The model under review builds one solid part; all positions refer to its coordinate system, in mm. A direction names the side the tool comes from. Round coordinates to 2 decimals unless told otherwise and drop trailing zeros. Loops run counter-clockwise (first coordinate to the right, second up) from the corner with the lowest first, then second, coordinate; pieces in that order, holes last. Notation, with made-up numbers: M 43.25,68.5 L 81.25,68.5 A21 ccw 81.25,75.5 Z; hole C 41,2 d1. An arc over 180 degrees is marked long. One line per question, with ' | ' between items.
from build123d import *

# Parameters (mm, degrees)
CHAMFER1_SIZE = 0.508


with BuildPart() as part:
    # Sketch1 → Revolve2 (revolve)
    with BuildSketch(Plane(origin=(0, 0, 0), x_dir=(0, 0, -1), z_dir=(1, 0, 0))):
        Polygon((-17.6958, 0), (-17.6958, 1.5), (-16.4258, 1.5), (-16.4258, 1.4), (-15.9258, 1.4), (-15.9258, 1.5), (-12.7508, 1.5), (-12.7508, 1.75), (0, 1.75), (0, 0), align=None)
    revolve2 = revolve(axis=Axis((0, 0, 0.682962963), (0, 0, 1)))

    # Mirror1: Revolve2 across plane
    add(revolve2.mirror(Plane.XY))

    # Chamfer1
    chamfer1_edges = [part.edges().sort_by_distance(p)[0] for p in [
        (0, -1.5, -17.6958),
        (0, -1.5, 17.6958),
    ]]
    chamfer(chamfer1_edges, length=CHAMFER1_SIZE)


solid = part.part
1) Machinability: for faces 5 (the cylindrical face through (0.67, 1.617, 0.179)), 6 (the cylindrical face through (-0.07, -1.5, 14.32)), 7 (the cylindrical face through (-0.07, -1.5, -16.8)), which of the approach directions +Z, -Z, +X, -X, +Y, -Y give a long, thin tool a straight path to every point of the face, cutting with its end or side? Answer none if there is none.
Output values:
face 5: +Z, -Z | face 6: +Z | face 7: -Z
2) For line 1 (Z direction, x = 0.7, y = 1.5); line 2 (Y direction, x = -0.1, z = 3); line 3 (X direction, y = -0.9, z = -7), list the stretches that pass through material, from the lowest coordinate up.
Output values:
line 1: z = -12.75 to 12.75 | line 2: y = -1.75 to 1.75 | line 3: x = -1.5 to 1.5
3) Add section C-C on z = -4. State the section outline as (x, y) points.
Output values:
outline: C 0,0 d3.5
4) Mouldability with a two-part tool opening along Z and no side actions: class faces 1 (the cylindrical face through (-0.06, -1.4, 16.17)), 2 (the cylindrical face through (-0.07, -1.5, -14.32)), 3 (the cylindrical face through (-0.06, -1.4, -16.17)), 4 (the flat face through (0, 0, 17.696)) as +Z half, -Z half, draft (parallel to the pull), parting line (faces both ways), or undercut.
Output values:
face 1: undercut | face 2: draft | face 3: undercut | face 4: +Z half
